Geometry: final body of the model. Coordinates: model frame, mm. A direction names the side the tool comes from. Round coordinates to 2 decimals unless told otherwise and drop trailing zeros. Order: outer loops, then holes, each group sorted by start corner. A loop starts at its lowest first (then second) coordinate and runs counter-clockwise, first axis right, second up. Notation, with made-up numbers: M 4,-22.75 L 29,-22.75 A21 cw 29,-4.75 Z; hole C 14,-34.5 d3. An arc over 180 degrees is marked long. Return JSON: item names as keys, results as strings. Group by question number.
Q1. Cut plane B-B on y = -9.5. Output: boundary loops of the cut face in (x, z), and give its area (3 significant figures).
Q2. Cut plane C-C on x = -10. Output: boundary loops of the cut face in (y, z), and give its area (3 significant figures).
Q3. Ray query, probe 1 along Y at (x, z) = (-10, 26.5); probe 2 along Z at (x, y) = (0, 33); probe 3 along X at (y, z) = (12.5, 6). Return the intervals inside material, ascending.
Q4. Mould query, pull axis Z, two halves, no side actions, for faces 1 (the face through (0.759, -32.465, 6.583)), 2 (the face through (30, 0, 30)), 3 (the face through (-27, 0, 0)). Classes: released by +Z, released by -Z, zero draft, split by the parting line, or undercut.
Q5. Cut plane D-D on z = 26.5. Output: boundary loops of the cut face in (x, y).
Q6. Access query for faces 4 (the face through (23, -29, 30)), 5 (the face through (0, 35, 30)). Directions: +Z, -Z, +X, -X, +Y, -Y. A direction counts if a zero-diameter tool reaches every point of the face in a straight line with its end or side. Return the directions, or none.
Q7. Cut plane A-A on x = 0. Output: boundary loops of the cut face in (y, z), and give its area (3 significant figures).
```python
from build123d import *

# Parameters (mm, degrees)
F0_W     = 60
F0_H     = 70
F0_W_2   = 50
F0_H_2   = 60
F1_DEPTH = 60
F2_R     = 5
F3_R     = 3.5
F4_DEPTH = 70


with BuildPart() as f1:
    # F0 (on Top) → F1 (new body)
    with BuildSketch(Plane.XY):
        Rectangle(F0_W, F0_H)
        Rectangle(F0_W_2, F0_H_2, mode=Mode.SUBTRACT)
    extrude(amount=F1_DEPTH)

    # F2
    f2_edges = [f1.edges().sort_by_distance(p)[0] for p in [
        (-30, 35, 30),
        (-30, -35, 30),
        (30, -35, 30),
        (30, 35, 30),
        (-25, -30, 30),
        (25, -30, 30),
        (25, 30, 30),
        (-25, 30, 30),
    ]]
    fillet(f2_edges, radius=F2_R)

    # F3 (on face) → F4 (cut)
    with BuildSketch(Plane(origin=(0, 35, 0), x_dir=(-1, 0, 0), z_dir=(0, 1, 0))):
        with Locations((0, 10)):
            Circle(F3_R)
    extrude(amount=-F4_DEPTH, mode=Mode.SUBTRACT)


solid = f1.part
```
Result sheet:
{
 "1": {"outline": "M -30,0 L -25,0 L -25,60 L -30,60 Z; M 25,0 L 30,0 L 30,60 L 25,60 Z", "area": "600 mm²"},
 "2": {"outline": "M -35,0 L -30,0 L -30,60 L -35,60 Z; M 30,0 L 35,0 L 35,60 L 30,60 Z", "area": "600 mm²"},
 "3": {"probe 1": "y = -35 to -30, 30 to 35", "probe 2": "z = 0 to 6.5, 13.5 to 60", "probe 3": "x = -30 to -25, 25 to 30"},
 "4": {"face 1": "undercut", "face 2": "zero draft", "face 3": "released by -Z"},
 "5": {"outline": "M -30,-30 A5 ccw -25,-35 L 25,-35 A5 ccw 30,-30 L 30,30 A5 ccw 25,35 L -25,35 A5 ccw -30,30 Z; hole M -25,-25 A5 ccw -20,-30 L 20,-30 A5 ccw 25,-25 L 25,25 A5 ccw 20,30 L -20,30 A5 ccw -25,25 Z"},
 "6": {"face 4": "+Z, -Z", "face 5": "+Z, -Z, +X, -X, +Y"},
 "7": {"outline": "M -35,0 L -30,0 L -30,6.5 L -35,6.5 Z; M -35,13.5 L -30,13.5 L -30,60 L -35,60 Z; M 30,0 L 35,0 L 35,6.5 L 30,6.5 Z; M 30,13.5 L 35,13.5 L 35,60 L 30,60 Z", "area": "530 mm²"}
}
